```python
from build123d import *

# Parameters (mm, degrees)
F0_W     = 914.4
F0_H     = 304.8
F1_DEPTH = 76.2
F1_TAPER = 3
F2_R     = 19.05
F3_T     = 6.35
F4_R     = 88.9
F5_DEPTH = 76.2010001


# Not quite as in the source:
# - a shell that OpenCascade refuses in one call is made with other operations: the cavity is built on its own and cut out


with BuildPart() as f1:
    # F0 (on Front) → F1 (new body)
    with BuildSketch(Plane.XZ):
        Rectangle(F0_W, F0_H)
    extrude(amount=F1_DEPTH, taper=F1_TAPER)

    # F2
    f2_edges = [f1.edges().sort_by_distance(p)[0] for p in [
        (455.203264, -38.1, 150.403264),
        (0, -76.2, 148.406527),
        (453.206527, -76.2, 0),
        (455.203264, -38.1, -150.403264),
        (0, -76.2, -148.406527),
        (-455.203264, -38.1, 150.403264),
        (-453.206527, -76.2, 0),
        (-455.203264, -38.1, -150.403264),
    ]]
    fillet(f2_edges, radius=F2_R)

    # F3: shell of thickness 6.35, made by hand


with BuildPart() as f3_core1:
    # F3_t2: copy of F1
    add(f1.part)

    # the walls: a layer under each face that stays
    f3_faces = [f3_core1.faces().sort_by_distance(p)[0] for p in [
        (0, -29.0734999832, 150.8763224299),
        (450.0967392281, -29.2790219143, 145.2967392281),
        (-450.0967392281, -29.2790219142, 145.2967392281),
        (0, -70.9683817678, 143.4419068897),
        (455.6763224299, -29.0734999832, 0),
        (-455.6763224299, -29.0734999832, 0),
        (450.0967392281, -29.2790219142, -145.2967392281),
        (-450.0967392281, -29.2790219142, -145.2967392281),
        (0, -29.0734999832, -150.8763224299),
        (444.4011528131, -70.968381766, 139.6011528105),
        (-448.0884256524, -67.5999269998, 139.5887948951),
        (0, -76.2, 0),
        (448.2419068897, -70.9683817678, 0),
        (-448.2419068897, -70.9683817678, 0),
        (444.388794687, -67.5999269998, -143.2884258011),
        (-448.0884256897, -67.5999270772, -139.5887947556),
        (0, -70.9683817678, -143.4419068897),
    ]]
    thicken(f3_faces, amount=-F3_T, mode=Mode.SUBTRACT)


with BuildPart() as f1_1:
    add(f1.part)

    # what is left inside the walls is the cavity
    f3_cavity = [f3_core1.part.solids().sort_by_distance(p)[0] for p in [
        (29.280349, -0.0635, -87.84086),
    ]]
    add(f3_cavity, mode=Mode.SUBTRACT)

    # F4 (on face) → F5 (cut, through all)
    with BuildSketch(Plane.XZ.offset(76.2)):
        with Locations((266.7, 0)):
            Circle(F4_R)
        Circle(F4_R)
        with Locations((-266.7, 0)):
            Circle(F4_R)
    extrude(amount=-F5_DEPTH, mode=Mode.SUBTRACT)


solid = f1_1.part
```
Work out the finished part from the listing and answer in its coordinate system (mm). A direction names the side the tool comes from. Give positions to 0.01 mm unless a question says otherwise; leave off trailing zeros.
(1) The part is cut by section A-A on z = 0. Count the separate pieces of the cut face and the enclosed holes in it, plus the area to 3 significant figures.
Final values:
separate pieces: 4
enclosed holes: 0
area: 3,180 mm2
(2) Which of the six approach directions +Z, -Z, +X, -X, +Y, -Y give full straight-line access (tool end or side, diameter ignored) to faces 3 (the flat face through (-6.134, -29.312, -144.505)), 4 (the flat face through (59, -76.2, -80))?
Final values:
face 3: +Y
face 4: +Z, -Z, +X, -X, -Y
(3) Flat-ended cylindrical pins translate along their axes: pin 1 Ø1.5 at (y, z) = (-33, 9.5) entering from -X; pin 2 Ø8 at (x, z) = (315, -75) entering from +Y; pin 3 Ø4 at (y, z) = (-51, -13) entering from -X. Find the tip coordinate at first contact, or state that the pin passes through.
Final values:
pin 1: stops at x = -455.51
pin 2: stops at y = -69.85
pin 3: stops at x = -454.63
(4) Straight lines are drawn through the part: line 1 (Z direction, x = 0, y = -71.5); line 2 (X direction, y = -72, z = 55); line 3 (Z direction, x = -417, y = -55). For each, find the intervals that lie inside material, in ascending order.
Final values:
line 1: z = -142.86 to -88.9, 88.9 to 142.86
line 2: x = -447.06 to -336.54, -196.86 to -69.84, 69.84 to 196.86, 336.54 to 447.06
line 3: z = -149.52 to -143.16, 143.16 to 149.52
(5) The mould has two halves that part along X. Classify faces 1 (the cylindrical face through (84.795, -73.069, 26.703)), 2 (the flat face through (11, 0, -150)): pulls with the +X half, pulls with the -X half, needs draft (parallel to the pull), parting line crosses it, or undercut.
Final values:
face 1: undercut
face 2: needs draft
